Input: part model. Units: mm. Frame: model coordinates. A direction names the side the tool comes from. Give positions to 0.01 mm unless a question says otherwise; leave off trailing zeros. Loops run counter-clockwise (first coordinate to the right, second up) from the corner with the lowest first, then second, coordinate; pieces in that order, holes last. Notation, with made-up numbers: M -11.75,88.25 L 47.25,88.25 A21 cw 47.25,105.25 Z; hole C -3,32 d1. An arc over 180 degrees is marked long. Answer as a JSON object with one key per item and string values. Group by question number.
1) Section query A-A on z = 1.5. Count the separate pieces of the cut face and the enclosed holes in it, plus the area to 3 significant figures.
2) Section query B-B on x = -19. Return loops of the section in (y, z), plus the area to 3 significant figures.
3) First-contact query: P1, Ø1.4, axis at x = -29.5, y = -2.5, coming from the +Z side; P2, Ø0.5, axis at x = -6, y = -2.5, coming from the +Z side. Flat tips, straight axial feed; report the tip coordinate or a pass-through.
4) Ray query, L1, parallel to Z at x = -19, y = -4.45. Return the intervals inside material, ascending.
5) Draft query along X for faces 1 (the flat face through (-8.5, -2.5, 1.5)), 2 (the flat face through (-18, -5, 1)), 3 (the flat face through (-35.7, -2, 1)). Return one class per face: +X half, -X half, draft (parallel to the pull), parting line (faces both ways), or undercut.
6) Access query for faces 4 (the flat face through (-13, -3, 1)), 5 (the flat face through (-11, -2, 2)). Directions: +Z, -Z, +X, -X, +Y, -Y. A direction counts if a zero-diameter tool reaches every point of the face in a straight line with its end or side. Return the directions, or none.
from build123d import *

# Parameters (mm, degrees)
F0_W     = 35.7
F0_H     = 2
F1_DEPTH = 5
F2_W     = 1.7
F2_H     = 1
F3_DEPTH = 5
F4_DEPTH = 5


with BuildPart() as f1:
    # F0 (on Front) → F1 (new body)
    with BuildSketch(Plane.XZ):
        with Locations((-17.85, 1)):
            Rectangle(F0_W, F0_H)
    extrude(amount=F1_DEPTH)

    # F2 (on face) → F3 (cut)
    with BuildSketch(Plane.XZ.offset(5)):
        with Locations((-33.15, 1.5)):
            Rectangle(F2_W, F2_H)
        with Locations((-29.75, 1.5)):
            Rectangle(F2_W, F2_H)
        with Locations((-26.35, 1.5)):
            Rectangle(F2_W, F2_H)
        with Locations((-22.95, 1.5)):
            Rectangle(F2_W, F2_H)
        with Locations((-19.55, 1.5)):
            Rectangle(F2_W, F2_H)
        with Locations((-16.15, 1.5)):
            Rectangle(F2_W, F2_H)
        with Locations((-12.75, 1.5)):
            Rectangle(F2_W, F2_H)
    extrude(amount=-F3_DEPTH, mode=Mode.SUBTRACT)

    # F2 (on face) → F4 (cut)
    with BuildSketch(Plane.XZ.offset(5)):
        with Locations((-9.35, 1.5)):
            Rectangle(F2_W, F2_H)
        with Locations((-5.95, 1.5)):
            Rectangle(F2_W, F2_H)
        with Locations((-2.55, 1.5)):
            Rectangle(F2_W, F2_H)
    extrude(amount=-F4_DEPTH, mode=Mode.SUBTRACT)


solid = f1.part
Output:
{
 "1": {"separate pieces": "11", "enclosed holes": "0", "area": "93.5 mm^2"},
 "2": {"outline": "M -5,0 L 0,0 L 0,1 L -5,1 Z", "area": "5.00 mm^2"},
 "3": {"P1": "stops at z = 2", "P2": "stops at z = 1"},
 "4": {"L1": "z = 0 to 1"},
 "5": {"face 1": "undercut", "face 2": "draft", "face 3": "-X half"},
 "6": {"face 4": "+Z, +Y, -Y", "face 5": "+Z, +X, -X, +Y, -Y"}
}
